```python
from build123d import *

# Parameters (mm, degrees)
ESBO_O2_W                  = 51
ESBO_O2_H                  = 50
RESSALTO_EXTRUS_O2_DEPTH   = 6
CORTE_EXTRUS_O1_DEPTH      = 25
CORTE_EXTRUS_O3_DEPTH      = 25
CORTE_EXTRUS_O5_DEPTH      = 37.067617785
CORTE_EXTRUS_O5_DEPTH_BACK = 37.067617785
ESBO_O5_R                  = 1.75
ESBO_O7_R                  = 1.5
CORTE_EXTRUS_O6_DEPTH      = 37.067617785


with BuildPart() as part:
    # Esbo_o2 → Ressalto-extrus_o2 (new body)
    with BuildSketch(Plane(origin=(0, 0, 0), x_dir=(1, 0, 0), z_dir=(0, 1, 0))):
        Rectangle(ESBO_O2_W, ESBO_O2_H)
    extrude(amount=RESSALTO_EXTRUS_O2_DEPTH)

    # Esbo_o3 → Corte-extrus_o1 (cut)
    with BuildSketch(Plane.XY.offset(25)):
        Polygon((-25.5, 0.6), (25.5, 5.06192184), (25.5, 6), (-25.5, 6), align=None)
    extrude(amount=-CORTE_EXTRUS_O1_DEPTH, mode=Mode.SUBTRACT)

    # Esbo_o4 → Corte-extrus_o3 (cut)
    with BuildSketch(Plane(origin=(0, 0, -25), x_dir=(-1, 0, 0), z_dir=(0, 0, -1))):
        Polygon((-25.5, 0.6), (25.5, 5.06192184), (25.5, 6), (-25.5, 6), align=None)
    extrude(amount=-CORTE_EXTRUS_O3_DEPTH, mode=Mode.SUBTRACT)

    # Esbo_o5 → Corte-extrus_o5 (cut, two sides: drawn at the far end of the back side and taken through both)
    with BuildSketch(Plane.XZ.offset(-CORTE_EXTRUS_O5_DEPTH_BACK)):
        with Locations(Location((0, 6, 0), (0, 0, 270))):
            Circle(ESBO_O5_R)
        with Locations(Location((0, 15, 0), (0, 0, 270))):
            Circle(ESBO_O5_R)
        with Locations(Location((0, -15, 0), (0, 0, 270))):
            Circle(ESBO_O5_R)
        with Locations(Location((0, -6, 0), (0, 0, 270))):
            Circle(ESBO_O5_R)
    extrude(amount=CORTE_EXTRUS_O5_DEPTH + CORTE_EXTRUS_O5_DEPTH_BACK, mode=Mode.SUBTRACT)

    # Esbo_o7 → Corte-extrus_o6 (cut, through all)
    with BuildSketch(Plane.XZ):
        with Locations(Location((-20, 20, 0), (0, 0, 270))):
            Circle(ESBO_O7_R)
        with Locations(Location((20, -20, 0), (0, 0, 270))):
            Circle(ESBO_O7_R)
    extrude(amount=-CORTE_EXTRUS_O6_DEPTH, mode=Mode.SUBTRACT)


solid = part.part
```
Model file for the job. Use its own axes, mm. A direction names the side the tool comes from. Give positions to 0.01 mm unless a question says otherwise; leave off trailing zeros. Write each loop counter-clockwise with the first axis right and the second up, starting at its lowest first coordinate (ties: lowest second). Pieces come first, ordered by that corner, then holes. Notation, with made-up numbers: (26, 38.5) - (82, 38.5) arc R22 ccw to (82, 69.5) - close; hole circle Ø5 at (4.5, -8.75). An arc over 180 degrees is marked (long way). One line per question, with ' | ' between items. Start each with the question number.
(1) Slice it at D-D on x = 20. Write the cut outline in (y, z), plus the area to 3 significant figures.
(2) 3-axis set-ups, long thin cutter, end or side, ignore diameter. For faces 4 (the face through (1.5, 1.5, 14.1)), 5 (the face through (-0.36, 2.8, 12.68)): which of +Z, -Z, +X, -X, +Y, -Y reach the whole face in a straight line?
(3) Slice it at A-A on z = 20. Write the cut outline in (x, y).
(4) Slice it at C-C on y = 1.85. Write the cut outline in (x, z), plus the area to 3 significant figures.
(5) Two-plate mould, pull along Z, no slides. Class faces 1 (the face through (-18.513, 0.611, 20.195)), 2 (the face through (0.36, 2.8, -12.68)), 3 (the face through (16, 3, 0)): +Z half, -Z half, draft (parallel to the pull), parting line (faces both ways), or undercut.
(6) Pin check, flat tips, straight feed: P1, Ø8, axis at x = 11.5, z = -8, coming from the +Y side; P2, Ø1.8, axis at x = 20, z = -20, coming from the +Y side; P3, Ø2, axis at x = 19.5, y = 3, coming from the -Z side; P4, Ø1.3, axis at x = -8, y = 3.5, coming from the +Z side. Stop position of each tip, or through.
(7) Wall check: line 1 along Z through (x, y) = (0, 1.1); line 2 along Z through (x, y) = (20, 0.7); line 3 along X through (y, z) = (0.4, -20). Give the ranges that are in metal, low to high. Write a range as from..to.
(8) Slice it at B-B on x = -1. Write the cut outline in (y, z).
Results below:
1) outline: (0, -25) - (1.08, -25) - (1.08, -21.5) - (0, -21.5) - close; (0, -18.5) - (1.08, -18.5) - (1.08, 0) - (4.58, 0) - (4.58, 25) - (0, 25) - close | area: 138 mm^2
2) face 4: +Y, -Y | face 5: +Z, -X, +Y
3) outline: (-25.5, 0) - (-21.5, 0) - (-21.5, 0.95) - (-25.5, 0.6) - close; (-18.5, 0) - (25.5, 0) - (25.5, 5.06) - (-18.5, 1.21) - close
4) outline: (-25.5, -25) - (11.21, -25) - (11.21, 0) - (25.5, 0) - (25.5, 25) - (-11.21, 25) - (-11.21, 0) - (-25.5, 0) - close; hole circle Ø3.5 at (0, -15); hole circle Ø3.5 at (0, -6); hole circle Ø3.5 at (0, 6); hole circle Ø3.5 at (0, 15) | area: 1,800 mm^2
5) face 1: undercut | face 2: draft | face 3: -Z half
6) P1: y = 2.17 | P2: through | P3: z = 0 | P4: z = 0
7) line 1: -25..-16.75, -13.25..-7.75, -4.25..4.25, 7.75..13.25, 16.75..25 | line 2: -25..-21.5, -18.5..25 | line 3: -25.5..18.5, 21.5..25.5
8) outline: (0, -25) - (2.92, -25) - (2.92, -16.44) - (0, -16.44) - close; (0, -13.56) - (2.92, -13.56) - (2.92, -7.44) - (0, -7.44) - close; (0, -4.56) - (2.92, -4.56) - (2.92, 0) - (2.74, 0) - (2.74, 4.56) - (0, 4.56) - close; (0, 7.44) - (2.74, 7.44) - (2.74, 13.56) - (0, 13.56) - close; (0, 16.44) - (2.74, 16.44) - (2.74, 25) - (0, 25) - close
